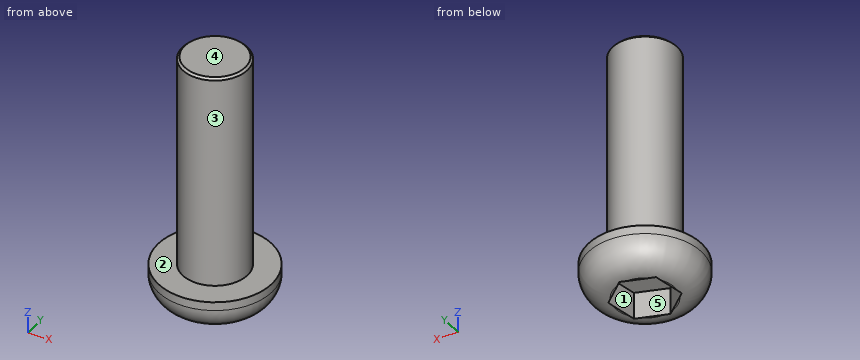
Autodesk Inventor part; units mm, degrees
ref_plane "YZ Plane" through (0, 0, 0) normal (1, 0, 0) x (0, 1, 0)
ref_plane "XZ Plane" through (0, 0, 0) normal (0, 1, 0) x (-1, 0, 0)
ref_plane "XY Plane" through (0, 0, 0) normal (0, 0, 1) x (1, 0, 0)
sketch "Sketch1" plane through (0, 0, 0) normal (0, 0, 1) x (1, 0, 0)
  circle A0 centre (0, 0) radius 3
  circle A1 centre (0, 0) radius 5.25
  dimension "d0" = 6
  dimension "d1" = 10.5
extrude "Extrusion1" add sketch "Sketch1" along normal blind 0.8
extrude "Extrusion2" add sketch "Sketch1" along normal blind 20.8 contours A0
thread "Thread1"
sketch "Boceto3" plane through (0, 0, 0) normal (0, 0, -1) x (-1, 0, 0)
  circle A0 centre (0, 0) radius 5.25
extrude "Extrusión3" add sketch "Boceto3" along normal blind 2.5
fillet "Empalme2" radius 2.5 1 edges at (5.25, 0, -2.5)
sketch "Boceto4" plane through (0, 0, -2.5) normal (0, 0, -1) x (-1, 0, 0)
  line L0 (-2.2122, -1.978) -> (-2.8191, 0.9269)
  line L1 (-2.8191, 0.9269) -> (-0.6069, 2.9049)
  line L2 (-0.6069, 2.9049) -> (2.2122, 1.978)
  line L3 (2.2122, 1.978) -> (2.8191, -0.9269)
  line L4 (2.8191, -0.9269) -> (0.6069, -2.9049)
  line L5 (0.6069, -2.9049) -> (-2.2122, -1.978)
  point P0 (0, 0)
  point P1 (0, 0)
  dimension "d12" = 5.14
extrude "Extrusión4" cut sketch "Boceto4" against normal blind 2.5
chamfer "Chaflán1" distance 0.2 angle 45 1 edges at (-3, 0, 20.8)
properties part number "Tornillo Allen cabeza botón M6x20mm"
The model under review builds one solid part; all positions refer to its coordinate system, in mm. Face numbers are marked on the shaded views. A direction names the side the tool comes from. Coordinates: 2 decimals unless noted, no trailing zeros. Write each loop counter-clockwise with the first axis right and the second up, starting at its lowest first coordinate (ties: lowest second). Pieces come first, ordered by that corner, then holes. Notation, with made-up numbers: (23.5, -27) - (39.5, -27) arc R7 ccw to (39.5, -20) - close; hole circle Ø2 at (66, -29). An arc over 180 degrees is marked (long way). Answer as a JSON object with one key per item and string values. Group by question number.
1. To check wall thickness, follow probe 1 along Y at (x, z) = (0, 12.5); probe 2 along Z at (x, y) = (-1, 0); probe 3 along Y at (x, z) = (-2.25, 16.5). State the ranges of each line that lie inside material, in increasing order.
2. Mouldability with a two-part tool opening along Y and no side actions: class the marked faces 1, 2 and 3 as pulls with the +Y half, pulls with the -Y half, needs draft (parallel to the pull), parting line crosses it, or undercut.
3. Add section A-A (y = 0). Give the boundary of the cut face in (x, z).
4. Machinability: for the marked faces 4 and 5, which of the approach directions +Z, -Z, +X, -X, +Y, -Y give a long, thin tool a straight path to every point of the face, cutting with its end or side? Answer none if there is none.
5. Add section B-B (z = 16). Give the boundary of the cut face in (x, y).
6. Clearance check with flat-ended pins moving along their axes: pin 1 Ø2 at (y, z) = (-2.5, 11) entering from +X; pin 2 Ø5 at (y, z) = (1.5, 12) entering from +X; pin 3 Ø1.7 at (x, y) = (-1, 1) entering from -Z. State where each tip first meets the part, or that it passes through.
Findings:
{
 "1": {"probe 1": "-3 to 3", "probe 2": "0 to 20.8", "probe 3": "-1.98 to 1.98"},
 "2": {"face 1": "undercut", "face 2": "needs draft", "face 3": "parting line crosses it"},
 "3": {"outline": "(-5.25, 0) arc R2.5 ccw to (-2.75, -2.5) - (-2.63, -2.5) - (-2.63, 0) - (2.63, 0) - (2.63, -2.5) - (2.75, -2.5) arc R2.5 ccw to (5.25, 0) - (5.25, 0.8) - (3, 0.8) - (3, 20.6) - (2.8, 20.8) - (-2.8, 20.8) - (-3, 20.6) - (-3, 0.8) - (-5.25, 0.8) - close"},
 "4": {"face 4": "+Z, +X, -X, +Y, -Y", "face 5": "-Z"},
 "5": {"outline": "circle Ø6 at (0, 0)"},
 "6": {"pin 1": "x = 2.6", "pin 2": "x = 3", "pin 3": "z = 0"}
}
